from build123d import *

# Parameters (mm, degrees)
SKETCH1_R                 = 16.891
SKETCH1_R_2               = 2.2479
BOSS_EXTRUDE1_DEPTH       = 3.175
TAP_DRILL_FOR_4_40_TAP1_D = 13.589
TAP_DRILL_FOR_2_56_TAP1_D = 1.778
CIRPATTERN1_COUNT         = 6


with BuildPart() as part:
    # Sketch1 → Boss-Extrude1 (new body)
    with BuildSketch(Plane.XY):
        Circle(SKETCH1_R)
        with Locations((0, -13.4874)):
            Circle(SKETCH1_R_2, mode=Mode.SUBTRACT)
        with Locations((-11.680431031, -6.7437)):
            Circle(SKETCH1_R_2, mode=Mode.SUBTRACT)
        with Locations((-11.680431031, 6.7437)):
            Circle(SKETCH1_R_2, mode=Mode.SUBTRACT)
        with Locations((0, 13.4874)):
            Circle(SKETCH1_R_2, mode=Mode.SUBTRACT)
        with Locations((11.680431031, 6.7437)):
            Circle(SKETCH1_R_2, mode=Mode.SUBTRACT)
        with Locations((11.680431031, -6.7437)):
            Circle(SKETCH1_R_2, mode=Mode.SUBTRACT)
    extrude(amount=BOSS_EXTRUDE1_DEPTH)

    # Tap Drill for #4-40 Tap1 (through all)
    with Locations(Plane.XY.offset(3.175)):
        with Locations((0, 0)):
            Hole(TAP_DRILL_FOR_4_40_TAP1_D / 2)

    # Tap Drill for #2-56 Tap1 (through all)
    with Locations(Plane.XY.offset(3.175)):
        with Locations((13.4874, 0)):
            tap_drill_for_2_56_tap1 = Hole(TAP_DRILL_FOR_2_56_TAP1_D / 2)

    # CirPattern1: Tap Drill for #2-56 Tap1 ×6 about axis
    cirpattern1_axis = Axis((0, 0, 0), (0, 0, 1))
    for i in range(1, CIRPATTERN1_COUNT):
        add(tap_drill_for_2_56_tap1.rotate(cirpattern1_axis, i * 360 / CIRPATTERN1_COUNT), mode=Mode.SUBTRACT)


solid = part.part
Build history of the part. All positions in model axes, mm. Coordinates: 2 decimals unless noted, no trailing zeros. Order: outer loops, then holes, each group sorted by start corner. A loop starts at its lowest first (then second) coordinate and runs counter-clockwise, first axis right, second up. Notation, with made-up numbers: (-1, 12) - (15, 12) arc R27 cw to (15, 46) - close; hole circle Ø10 at (-31, 7). An arc over 180 degrees is marked (long way). Write item = value, one per line. Start each with the question number.
1) Saw through at A-A on x = 0. Write the cut outline in (y, z) (1 decimal).
2) Saw through at D-D on z = 2.2. Count the separate pieces of the cut face and the enclosed holes in it, then the cut area to 3 significant figures.
3) Saw through at B-B on y = 7.5. Write the cut outline in (x, z) (3 decimals).
4) Wall check: line 1 along Y through (x, z) = (0, 1.85); line 2 along Y through (x, z) = (-12, 3); line 3 along X through (y, z) = (12, 2.9). Give the ranges that are in metal, low to high. Write a range as from..to.
5) Flat gauge pins, fed straight in: pin 1 Ø1.1 at (x, y) = (-13.49, 0) entering from -Z; pin 2 Ø1.5 at (y, z) = (-6, 0.5) entering from +X. Where does each tip first touch, or does it go through?
6) Two-plate mould, pull along Y, no slides. Class faces 1 (the face through (16.111, 5.074, 1.565)), 2 (the face through (0, -7, 0)), 3 (the face through (6.628, -12.562, 1.565)), 4 (the face through (-7.22, 12.43, 1.57)): pulls with the +Y half, pulls with the -Y half, needs draft (parallel to the pull), parting line crosses it, or undercut.
7) Saw through at C-C on x = -12. Write the cut outline in (y, z) (3 decimals), then the cut area to 3 significant figures.
From the geometry:
q1.outline = (-16.9, 0) - (-15.7, 0) - (-15.7, 3.2) - (-16.9, 3.2) - close; (-11.2, 0) - (-6.8, 0) - (-6.8, 3.2) - (-11.2, 3.2) - close; (6.8, 0) - (11.2, 0) - (11.2, 3.2) - (6.8, 3.2) - close; (15.7, 0) - (16.9, 0) - (16.9, 3.2) - (15.7, 3.2) - close
q2.separate_pieces = 1
q2.enclosed_holes = 13
q2.area = 641 mm^2
q3.outline = (-15.135, 0) - (-13.797, 0) - (-13.797, 3.175) - (-15.135, 3.175) - close; (-9.564, 0) - (9.564, 0) - (9.564, 3.175) - (-9.564, 3.175) - close; (13.797, 0) - (15.135, 0) - (15.135, 3.175) - (13.797, 3.175) - close
q4.line_1 = -16.89..-15.74, -11.24..-6.79, 6.79..11.24, 15.74..16.89
q4.line_2 = -11.89..-8.97, -4.52..4.52, 8.97..11.89
q4.line_3 = -11.89..-7.57, -5.91..-1.69, 1.69..5.91, 7.57..11.89
q5.pin_1 = through
q5.pin_2 = 16.05
q6.face_1 = parting line crosses it
q6.face_2 = needs draft
q6.face_3 = undercut
q6.face_4 = undercut
q7.outline = (-11.887, 0) - (-8.969, 0) - (-8.969, 3.175) - (-11.887, 3.175) - close; (-4.519, 0) - (4.519, 0) - (4.519, 3.175) - (-4.519, 3.175) - close; (8.969, 0) - (11.887, 0) - (11.887, 3.175) - (8.969, 3.175) - close
q7.area = 47.2 mm^2
